from build123d import *

# Parameters (mm, degrees)
SKETCH1_W           = 91
SKETCH1_H           = 28
BOSS_EXTRUDE1_DEPTH = 17.5
SKETCH2_R           = 4
CUT_EXTRUDE1_DEPTH  = 0.5
SKETCH3_R           = 2
CUT_EXTRUDE2_DEPTH  = 6.5
FILLET1_R           = 3


with BuildPart() as part:
    # Sketch1 → Boss-Extrude1 (new body)
    with BuildSketch(Plane(origin=(0, 0, 0), x_dir=(1, 0, 0), z_dir=(0, 1, 0))):
        with Locations((45.5, 14)):
            Rectangle(SKETCH1_W, SKETCH1_H)
    extrude(amount=BOSS_EXTRUDE1_DEPTH)

    # Sketch2 → Cut-Extrude1 (cut)
    with BuildSketch(Plane(origin=(0, 17.5, 0), x_dir=(1, 0, 0), z_dir=(0, 1, 0))):
        with Locations((45.5, 19)):
            Circle(SKETCH2_R)
        with Locations((8, 19)):
            Circle(SKETCH2_R)
        with Locations((83, 19)):
            Circle(SKETCH2_R)
    extrude(amount=-CUT_EXTRUDE1_DEPTH, mode=Mode.SUBTRACT)

    # Sketch3 → Cut-Extrude2 (cut)
    with BuildSketch(Plane.XZ):
        with Locations((83, -18.5)):
            Circle(SKETCH3_R)
        with Locations((8, -18.5)):
            Circle(SKETCH3_R)
    extrude(amount=-CUT_EXTRUDE2_DEPTH, mode=Mode.SUBTRACT)

    # Fillet1
    fillet1_edges = [part.edges().sort_by_distance(p)[0] for p in [
        (0, 8.75, -28),
        (91, 8.75, -28),
        (91, 8.75, 0),
        (0, 8.75, 0),
    ]]
    fillet(fillet1_edges, radius=FILLET1_R)


solid = part.part
The model under review builds one solid part; all positions refer to its coordinate system, in mm. A direction names the side the tool comes from. Give positions to 0.01 mm unless a question says otherwise; leave off trailing zeros. Order: outer loops, then holes, each group sorted by start corner. A loop starts at its lowest first (then second) coordinate and runs counter-clockwise, first axis right, second up. Notation, with made-up numbers: M 84,-25.5 L 103,-25.5 A28 cw 103,12.5 Z; hole C -26,84 d2. An arc over 180 degrees is marked long. Use one line per item in the form item = value. Start each with the question number.
Item 1: For faces 4 (the cylindrical face through (84.908, 3.204, -17.899)), 5 (the flat face through (8, 17, -19)), 6 (the cylindrical face through (90.1, 8.87, -27.14)), list the 3-axis set-ups (+Z, -Z, +X, -X, +Y, -Y) from which the entire face can be reached by the end or side of a thin tool; tool diameter is ignored.
Item 2: To check wall thickness, follow line 1 along X through (y, z) = (17.45, -19); line 2 along Z through (x, y) = (83, 5.25); line 3 along Z through (x, y) = (8, 17.3). State the ranges of each line that lie inside material, in increasing order. Write a range as from..to.
Item 3: We need section A-A on x = 83. Give the boundary of the cut face in (y, z), plus the area to 3 significant figures.
Item 4: The part is to be moulded in two halves that separate along X. For faces 1 (the cylindrical face through (7.74, 3.204, -16.517)), 2 (the cylindrical face through (90.1, 8.87, -0.86)), 3 (the flat face through (45, 0, -14)), say which applies: pulls with the +X half, pulls with the -X half, needs draft (parallel to the pull), parting line crosses it, or undercut.
Item 5: Insertion check: pin 1 Ø1.2 at (x, z) = (83, -19) entering from -Y; pin 2 Ø4 at (x, z) = (7, -20) entering from +Y. Each pin has a flat end and moves straight along its axis. Give the tip position at first contact, or say it passes through.
Completed:
q1.face_4 = -Y
q1.face_5 = +Y
q1.face_6 = -Z, +X, +Y, -Y
q2.line_1 = 0..4, 12..41.5, 49.5..79, 87..91
q2.line_2 = -28..-20.5, -16.5..0
q2.line_3 = -28..-23, -15..0
q3.outline = M 0,-28 L 17.5,-28 L 17.5,-23 L 17,-23 L 17,-15 L 17.5,-15 L 17.5,0 L 0,0 L 0,-16.5 L 6.5,-16.5 L 6.5,-20.5 L 0,-20.5 Z
q3.area = 460 mm²
q4.face_1 = undercut
q4.face_2 = pulls with the +X half
q4.face_3 = needs draft
q5.pin_1 = 6.5
q5.pin_2 = 17
